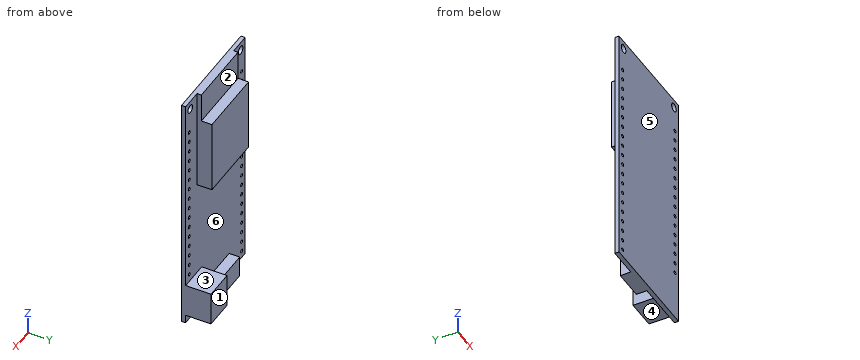
Autodesk Inventor part; units mm, degrees
ref_plane "YZ Plane" through (0, 0, 0) normal (1, 0, 0) x (0, 1, 0)
ref_plane "XZ Plane" through (0, 0, 0) normal (0, 1, 0) x (-1, 0, 0)
ref_plane "XY Plane" through (0, 0, 0) normal (0, 0, 1) x (1, 0, 0)
sketch "Эскиз1" plane through (0, 0, 0) normal (0, 1, 0) x (-1, 0, 0)
  line L0 (0, 0) -> (26, 0)
  line L1 (26, 0) -> (26, -58)
  line L2 (26, -58) -> (0, -58)
  line L3 (0, -58) -> (0, 0)
  dimension "d0" = 58
  dimension "d1" = 26
extrude "Выдавливание1" add sketch "Эскиз1" along normal blind 1
sketch "Эскиз2" plane through (0, 1, 0) normal (0, 1, 0) x (1, 0, 0)
  line L0 (-26, 0) -> (0, 0)
  line L1 (-26, 58) -> (-26, 0)
  line L2 (0, 0) -> (0, 58)
  point P0 (-24, 2)
  point P1 (-2, 2)
  dimension "d4" = 2
  dimension "d5" = 2
  dimension "d6" = 2
  dimension "d7" = 2
hole "Отверстие1" at (-24, 1, -2) at (-2, 1, -2) direction (0, -1, 0) diameter 2 end through all
sketch "Эскиз3" plane through (0, 1, 0) normal (0, 1, 0) x (1, 0, 0)
  line L0 (-12, 53) -> (-19, 53)
  line L1 (-19, 53) -> (-19, 58)
  line L2 (-19, 58) -> (-12, 58)
  line L3 (-12, 58) -> (-12, 53)
  line L4 (0, 58) -> (-26, 58)
  line L5 (-26, 58) -> (-26, 0)
  point P0 (0, 0)
  dimension "d15" = 7
  dimension "d16" = 5
  dimension "d17" = 7
extrude "Выдавливание2" add sketch "Эскиз3" along normal blind 2.5
sketch "Эскиз4" plane through (0, 1, 0) normal (0, 1, 0) x (1, 0, 0)
  line L0 (-7, 48) -> (0, 48)
  line L1 (0, 48) -> (0, 56)
  line L2 (0, 56) -> (-7, 56)
  line L3 (-7, 56) -> (-7, 48)
  line L4 (0, 0) -> (0, 58)
  line L5 (0, 58) -> (-12, 58)
  dimension "d20" = 7
  dimension "d21" = 8
  dimension "d22" = 2
extrude "Выдавливание3" add sketch "Эскиз4" along normal blind 6
sketch "Эскиз5" plane through (0, 1, 0) normal (0, 1, 0) x (1, 0, 0)
  line L0 (-21, 7) -> (-5, 7)
  line L1 (-5, 7) -> (-5, 24.5)
  line L2 (-5, 24.5) -> (-21, 24.5)
  line L3 (-21, 24.5) -> (-21, 7)
  line L4 (-26, 0) -> (0, 0)
  point P0 (-13, 7)
  point P1 (-13, 0)
  dimension "d25" = 17.5
  dimension "d26" = 16
  dimension "d27" = 7
extrude "Выдавливание4" add sketch "Эскиз5" along normal blind 3.5
sketch "Эскиз6" plane through (0, 1, 0) normal (0, 1, 0) x (1, 0, 0)
  line L0 (-5, 7) -> (-21, 7)
  line L1 (-5, 7) -> (-21, 7)
  line L2 (-21, 7) -> (-21, 0)
  line L3 (-21, 0) -> (-5, 0)
  line L4 (-5, 0) -> (-5, 7)
  line L5 (-21, 24.5) -> (-21, 7)
  line L6 (-26, 0) -> (0, 0)
extrude "Выдавливание5" add sketch "Эскиз6" along normal blind 1
sketch "Эскиз7" plane through (0, 1, 0) normal (0, 1, 0) x (1, 0, 0)
  line L0 (-26, 0) -> (-21, 0)
  line L1 (-26, 58) -> (-26, 0)
  line L2 (0, 0) -> (0, 48)
  point P0 (-24.43, 8)
  point P1 (-24.43, 10.54)
  point P2 (-24.43, 13.08)
  point P3 (-24.43, 15.62)
  point P4 (-24.43, 18.16)
  point P5 (-24.43, 20.7)
  point P6 (-24.43, 23.24)
  point P7 (-24.43, 25.78)
  point P8 (-24.43, 28.32)
  point P9 (-24.43, 30.86)
  point P10 (-24.43, 33.4)
  point P11 (-24.43, 35.94)
  point P12 (-24.43, 38.48)
  point P13 (-24.43, 41.02)
  point P14 (-24.43, 43.56)
  point P15 (-24.43, 46.1)
  point P16 (-24.43, 48.64)
  point P17 (-24.43, 51.18)
  point P18 (-24.43, 53.72)
  point P19 (-24.43, 56.26)
  point P20 (-1.57, 8)
  point P21 (-1.57, 10.54)
  point P22 (-1.57, 13.08)
  point P23 (-1.57, 15.62)
  point P24 (-1.57, 18.16)
  point P25 (-1.57, 20.7)
  point P26 (-1.57, 23.24)
  point P27 (-1.57, 25.78)
  point P28 (-1.57, 28.32)
  point P29 (-1.57, 30.86)
  point P30 (-1.57, 33.4)
  point P31 (-1.57, 35.94)
  point P32 (-1.57, 38.48)
  point P33 (-1.57, 41.02)
  point P34 (-1.57, 43.56)
  point P35 (-1.57, 46.1)
  dimension "d32" = 8
  dimension "d33" = 1.57
  dimension "d36" = 2.54
  dimension "d48" = 1.57
  dimension "d51" = 2.54
hole "Отверстие2" at (-24.43, 1, -8) at (-24.43, 1, -10.54) at (-24.43, 1, -13.08) at (-24.43, 1, -15.62) at (-24.43, 1, -18.16) at (-24.43, 1, -20.7) at (-24.43, 1, -23.24) at (-24.43, 1, -25.78) at (-24.43, 1, -28.32) at (-24.43, 1, -30.86) at (-24.43, 1, -33.4) at (-24.43, 1, -35.94) at (-24.43, 1, -38.48) at (-24.43, 1, -41.02) at (-24.43, 1, -43.56) at (-24.43, 1, -46.1) at (-24.43, 1, -48.64) at (-24.43, 1, -51.18) at (-24.43, 1, -53.72) at (-24.43, 1, -56.26) at (-1.57, 1, -46.1) at (-1.57, 1, -43.56) at (-1.57, 1, -41.02) at (-1.57, 1, -38.48) at (-1.57, 1, -35.94) at (-1.57, 1, -33.4) at (-1.57, 1, -25.78) at (-1.57, 1, -23.24) at (-1.57, 1, -20.7) at (-1.57, 1, -18.16) at (-1.57, 1, -15.62) at (-1.57, 1, -13.08) at (-1.57, 1, -10.54) at (-1.57, 1, -28.32) at (-1.57, 1, -30.86) at (-1.57, 1, -8) direction (0, -1, 0) diameter 0.8 end through all
properties part number "ESP32 LOLIN32 V1.0.0"
Input: part model. Units: mm. Frame: model coordinates. Face numbers are marked on the shaded views. A direction names the side the tool comes from. Give positions to 0.01 mm unless a question says otherwise; leave off trailing zeros. Order: outer loops, then holes, each group sorted by start corner. A loop starts at its lowest first (then second) coordinate and runs counter-clockwise, first axis right, second up. Notation, with made-up numbers: M -26.5,32.5 L 13.5,32.5 A18 cw 13.5,51.5 Z; hole C -30,-24 d8. An arc over 180 degrees is marked long. One line per question, with ' | ' between items. Start each with the question number.
1. Pull-direction query (Z, two-part tool) for the marked faces 3, 4, 5 and 6; classes: released by +Z, released by -Z, zero draft, split by the parting line, or undercut.
2. Access query for the marked faces 1 and 2. Directions: +Z, -Z, +X, -X, +Y, -Y. A direction counts if a zero-diameter tool reaches every point of the face in a straight line with its end or side. Return the directions, or none.
3. Section query B-B (x = -9.5). Return the cut outline in (y, z).
4. Section query C-C (z = -35). Return the cut outline in (x, y), and give its area (3 significant figures).
5. First-contact query: pin 1 Ø2 at (x, y) = (-21, 2.5) entering from -Z; pin 2 Ø1.8 at (y, z) = (2.5, -10) entering from -X; pin 3 Ø3 at (x, y) = (-18, 4.5) entering from +Z. Flat tips, straight axial feed; report the tip coordinate or a pass-through.
6. Material intervals for probe 1 along X at (y, z) = (0.75, -43.56); probe 2 along Z at (x, y) = (-2, 5.75); probe 3 along X at (y, z) = (6.5, -55), sorted ascending. Write a range as [from, to].
7. Section query A-A (z = -2). Return the cut outline in (x, y), and give its area (3 significant figures).
Here are the results:
1) face 3: undercut | face 4: released by -Z | face 5: zero draft | face 6: undercut
2) face 1: +Z, -Z, +X, -X, +Y | face 2: +Z, +X, -X, +Y
3) outline: M 0,-58 L 1,-58 L 1,-24.5 L 4.5,-24.5 L 4.5,-7 L 2,-7 L 2,0 L 0,0 Z
4) outline: M -26,0 L 0,0 L 0,1 L -26,1 Z | area: 26.0 mm²
5) pin 1: z = -24.5 | pin 2: x = -21 | pin 3: z = -7
6) probe 1: [-26, -24.83], [-24.03, -1.97], [-1.17, 0] | probe 2: [-56, -48] | probe 3: [-7, 0]
7) outline: M -26,0 L -25,0 L -25,1 L -26,1 Z; M -23,0 L -3,0 L -3,1 L -5,1 L -5,2 L -21,2 L -21,1 L -23,1 Z; M -1,0 L 0,0 L 0,1 L -1,1 Z | area: 38.0 mm²
